Can you work these out from the model? Positions are in its coordinate system, mm. A direction names the side the tool comes from. Round coordinates to 2 decimals unless told otherwise and drop trailing zeros. Order: outer loops, then holes, each group sorted by start corner. A loop starts at its lowest first (then second) coordinate and runs counter-clockwise, first axis right, second up. Notation, with made-up numbers: (75, -12) -> (97, -12) arc R11 cw to (97, -1) -> close; hole circle Ø1 at (-18.75, -10). An arc over 180 degrees is marked (long way). One line per item, written item: value.
```python
from build123d import *

# Parameters (mm, degrees)
ESBO_O1_W                = 120
ESBO_O1_H                = 147
RESSALTO_EXTRUS_O1_DEPTH = 6
CORTE_EXTRUS_O1_DEPTH    = 96.069711265
ESBO_O3_W                = 6
ESBO_O3_H                = 6
CORTE_EXTRUS_O2_DEPTH    = 96.069711265
PADR_O_LINEAR1_COUNT     = 7
PADR_O_LINEAR1_PITCH     = 10.75
PADR_O_LINEAR1_COL_COUNT = 7
PADR_O_LINEAR1_COL_PITCH = 10.75
PADR_O_LINEAR2_COUNT     = 5
PADR_O_LINEAR2_PITCH     = 11.4
PADR_O_LINEAR3_COUNT     = 5
PADR_O_LINEAR3_PITCH     = 11.4
ESBO_O4_W                = 6
ESBO_O4_H                = 6
CORTE_EXTRUS_O3_DEPTH    = 96.069711265
PADR_O_LINEAR4_COUNT     = 5
PADR_O_LINEAR4_PITCH     = 11.4
PADR_O_LINEAR5_COUNT     = 5
PADR_O_LINEAR5_PITCH     = 11.4


with BuildPart() as part:
    # Esboço1 → Ressalto-extrusão1 (new body)
    with BuildSketch(Plane.XY):
        Rectangle(ESBO_O1_W, ESBO_O1_H)
    extrude(amount=RESSALTO_EXTRUS_O1_DEPTH)

    # Esboço2 → Corte-extrusão1 (cut, symmetric)
    with BuildSketch(Plane.XY.offset(6)):
        Polygon((-3, 403.362470446), (-3, 73.5), (-3, 67.5), (3, 67.5), (3, 73.5), (3, 403.362470446), (3, 1063.087411339), (-3, 1063.087411339), align=None)
    corte_extrus_o1 = extrude(amount=CORTE_EXTRUS_O1_DEPTH, both=True, mode=Mode.SUBTRACT)

    # Esboço3 → Corte-extrusão2 (cut, through all)
    with BuildSketch(Plane.XY.offset(6)):
        with Locations((-57, 0)):
            Rectangle(ESBO_O3_W, ESBO_O3_H)
        with Locations((57, 0)):
            Rectangle(ESBO_O3_W, ESBO_O3_H)
    corte_extrus_o2 = extrude(amount=-CORTE_EXTRUS_O2_DEPTH, mode=Mode.SUBTRACT)

    # Padrão linear1: Corte-extrusão2 ×7
    with Locations(*[(0, i * PADR_O_LINEAR1_PITCH, 0) for i in range(1, PADR_O_LINEAR1_COUNT)]):
        add(corte_extrus_o2, mode=Mode.SUBTRACT)

    # Padrão linear1 col: Corte-extrusão2 ×7
    with Locations(*[(0, -i * PADR_O_LINEAR1_COL_PITCH, 0) for i in range(1, PADR_O_LINEAR1_COL_COUNT)]):
        add(corte_extrus_o2, mode=Mode.SUBTRACT)

    # Padrão linear2: Corte-extrusão1 ×5
    with Locations(*[(-i * PADR_O_LINEAR2_PITCH, 0, 0) for i in range(1, PADR_O_LINEAR2_COUNT)]):
        add(corte_extrus_o1, mode=Mode.SUBTRACT)

    # Padrão linear3: Corte-extrusão1 ×5
    with Locations(*[(i * PADR_O_LINEAR3_PITCH, 0, 0) for i in range(1, PADR_O_LINEAR3_COUNT)]):
        add(corte_extrus_o1, mode=Mode.SUBTRACT)

    # Esboço4 → Corte-extrusão3 (cut, through all)
    with BuildSketch(Plane.XY.offset(6)):
        with Locations((0, -70.5)):
            Rectangle(ESBO_O4_W, ESBO_O4_H)
    corte_extrus_o3 = extrude(amount=-CORTE_EXTRUS_O3_DEPTH, mode=Mode.SUBTRACT)

    # Padrão linear4: Corte-extrusão3 ×5
    with Locations(*[(-i * PADR_O_LINEAR4_PITCH, 0, 0) for i in range(1, PADR_O_LINEAR4_COUNT)]):
        add(corte_extrus_o3, mode=Mode.SUBTRACT)

    # Padrão linear5: Corte-extrusão3 ×5
    with Locations(*[(i * PADR_O_LINEAR5_PITCH, 0, 0) for i in range(1, PADR_O_LINEAR5_COUNT)]):
        add(corte_extrus_o3, mode=Mode.SUBTRACT)


solid = part.part
```
Q1. Will these pins go through, and if not, where does the flat tip stop? pin 1 Ø3 at (x, z) = (-23, 4.5) entering from -Y; pin 2 Ø1 at (y, z) = (23.5, 2.5) entering from -X; pin 3 Ø1.8 at (y, z) = (20.5, 2.5) entering from +X.
Answers below:
pin 1: y = -67.5
pin 2: x = -54
pin 3: x = 54
Q2. I want a section at A-A on y = 31.5. List the corners of the cut face in (x, z) for me.
Answers below:
outline: (-54, 0) -> (54, 0) -> (54, 6) -> (-54, 6) -> close
Q3. On a 3-axis mill with a long thin cutter (end or side, diameter ignored), from which of +Z, -Z, +X, -X, +Y, -Y can I reach the whole of each face in a straight line? I mean faces 1 (the face through (-42.6, -71, 3)), 2 (the face through (57, -67.5, 3)), 3 (the face through (-54, 64, 3)). Say none if no direction works.
Answers below:
face 1: +Z, -Z, -Y
face 2: +Z, -Z, +X
face 3: +Z, -Z, -X
Q4. Please list where these lines run through material, in increasing order: line 1 along Y through (x, z) = (-47.5, 2.05); line 2 along X through (y, z) = (-41.5, 4.85).
Answers below:
line 1: -67.5 to 67.5
line 2: -54 to 54
Q5. We'd pull the mould along Y, two halves only. Please class faces 4 (the face through (-46, 67.5, 3)), 5 (the face through (-60, -5, 3)), 6 (the face through (-57, -50.75, 3)): released by +Y, released by -Y, zero draft, split by the parting line, or undercut.
Answers below:
face 4: released by +Y
face 5: zero draft
face 6: undercut
